```python
from build123d import *

# Parameters (mm, degrees)
SKETCH004_W  = 10
SKETCH004_H  = 8
PAD004_DEPTH = 1.15
SKETCH_R     = 4
PAD_DEPTH    = 4
SKETCH001_R  = 3.9
PAD001_DEPTH = 0.5
SKETCH002_R  = 4
PAD002_DEPTH = 9.5
SKETCH003_R  = 3.5
PAD003_DEPTH = 7.5
FILLET_R     = 1.5
FILLET001_R  = 0.499
FILLET002_R  = 0.099
SKETCH005_R  = 1.1
POCKET_DEPTH = 5


with BuildPart() as body001:
    # Sketch004 (on DatumPlane) → Pad004 (new body, symmetric)
    with BuildSketch(Plane(origin=(0, 0, 17), x_dir=(1, 0, 0), z_dir=(0, -1, 0))):
        with Locations((0, 1)):
            Rectangle(SKETCH004_W, SKETCH004_H)
    extrude(amount=PAD004_DEPTH, both=True)


with BuildPart() as body:
    # Sketch → Pad (new body)
    with BuildSketch(Plane.XY):
        Circle(SKETCH_R)
    extrude(amount=PAD_DEPTH)

    # Sketch001 (on Face3 of Pad) → Pad001 (join)
    with BuildSketch(Plane.XY.offset(4)):
        Circle(SKETCH001_R)
    extrude(amount=PAD001_DEPTH)

    # Sketch002 (on Face5 of Pad001) → Pad002 (join)
    with BuildSketch(Plane.XY.offset(4.5)):
        Circle(SKETCH002_R)
    extrude(amount=PAD002_DEPTH)

    # Sketch003 (on Face3 of Pad002) → Pad003 (join)
    with BuildSketch(Plane.XY.offset(14)):
        Circle(SKETCH003_R)
    extrude(amount=PAD003_DEPTH)

    # Fillet
    fillet_edges = [body.edges().sort_by_distance(p)[0] for p in [
        (-3.5, 0, 21.5),
    ]]
    fillet(fillet_edges, radius=FILLET_R)

    # Fillet001
    fillet001_edges = [body.edges().sort_by_distance(p)[0] for p in [
        (-4, 0, 14),
    ]]
    fillet(fillet001_edges, radius=FILLET001_R)

    # Fillet002
    fillet002_edges = [body.edges().sort_by_distance(p)[0] for p in [
        (-4, 0, 4),
        (-4, 0, 4.5),
    ]]
    fillet(fillet002_edges, radius=FILLET002_R)

    # Boolean: cut Body001
    add(body001.part, mode=Mode.SUBTRACT)

    # Sketch005 (on Face14 of Boolean) → Pocket (cut, symmetric)
    with BuildSketch(Plane.XZ.offset(-1.15)):
        with Locations((0, 18)):
            Circle(SKETCH005_R)
    extrude(amount=POCKET_DEPTH, both=True, mode=Mode.SUBTRACT)


solid = body.part
```
Model file for the job. Use its own axes, mm. A direction names the side the tool comes from. Give positions to 0.01 mm unless a question says otherwise; leave off trailing zeros. Loops run counter-clockwise (first coordinate to the right, second up) from the corner with the lowest first, then second, coordinate; pieces in that order, holes last. Notation, with made-up numbers: (33.25, 14.25) - (71.25, 14.25) arc R25 cw to (71.25, 49.25) - close; hole circle Ø1 at (60.5, 83). An arc over 180 degrees is marked (long way). One line per item, written item: value. Start each with the question number.
1. Probe L1, parallel to Z at x = 2.5, y = -0.25; L2, parallel to X at y = -2.05, z = 18; L3, parallel to Y at x = -1.25, z = 15. List the from-to ranges inside material, lowest first. Write a range as from..to.
2. Pin check, flat tips, straight feed: pin 1 (2.5 mm diameter, centred on x = 1.5, y = 0, fed in from +Z); pin 2 (3.5 mm diameter, centred on x = 0, z = 18, fed in from -Y); pin 3 (1.5 mm diameter, centred on y = -1, z = 11.5, fed in from +X); pin 4 (1.5 mm diameter, centred on x = 2, y = 0, fed in from +Z). Stop position of each tip, or through.
3. Slice it at C-C (x = 0). Give the number of separate pieces and of enclosed holes in the cut face, plus the area to 3 significant figures.
4. Pull direction Z, two halves, no side cores. Call faces 4 (the cylindrical face through (-0.867, -3.905, 8.988)), 5 (the cylindrical face through (-0.14, -2.34, 19.09)), 6 (the flat face through (0, -1.5, 21.5)): pulls with the +Z half, pulls with the -Z half, needs draft (parallel to the pull), parting line crosses it, or undercut.
5. Slice it at D-D (z = 15.5). List the corners of the cut face in (x, y), plus the area to 3 significant figures.
6. Slice it at B-B (z = 18). List the corners of the cut face in (x, y), plus the area to 3 significant figures.
7. Which spindle directions (+Z, -Z, +X, -X, +Y, -Y) get a long thin tool onto all of the face, cutting with end or side? Do faces 1 (the cylindrical face through (-0.1, -3.5, 16.3)), 2 (the cylindrical face through (-2.87, 2.64, 4.25)), 3 (the flat face through (1, 1.15, 17)). Say none if no direction does.
Solution:
1. L1: z = 0..14
1. L2: x = -2.84..-1.1, 1.1..2.84
1. L3: y = -3.27..-1.15, 1.15..3.27
2. pin 1: stops at z = 21.5
2. pin 2: stops at y = -3.5
2. pin 3: stops at x = 3.99
2. pin 4: stops at z = 14
3. separate pieces: 3
3. enclosed holes: 0
3. area: 136 mm^2
4. face 4: needs draft
4. face 5: undercut
4. face 6: pulls with the +Z half
5. outline: (-3.31, -1.15) arc R3.5 ccw to (3.31, -1.15) - close; (-3.31, 1.15) - (3.31, 1.15) arc R3.5 ccw to start
5. area: 22.7 mm^2
6. outline: (-3.31, -1.15) arc R3.5 ccw to (-1.1, -3.32) - (-1.1, -1.15) - close; (-3.31, 1.15) - (-1.1, 1.15) - (-1.1, 3.32) arc R3.5 ccw to start; (1.1, -3.32) arc R3.5 ccw to (3.31, -1.15) - (1.1, -1.15) - close; (1.1, 1.15) - (3.31, 1.15) arc R3.5 ccw to (1.1, 3.32) - close
6. area: 12.6 mm^2
7. face 1: +Z, -Y
7. face 2: none
7. face 3: +Z, +X, -X
